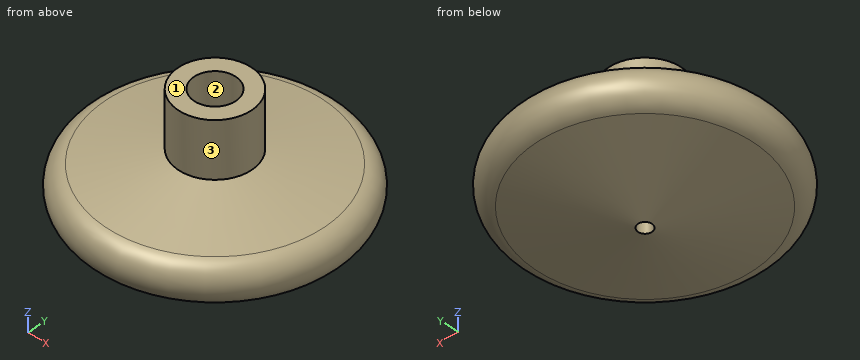
from build123d import *

# Parameters (mm, degrees)
F2_R     = 4.7625
F3_DEPTH = 9.525
F4_R     = 1.5875
F5_DEPTH = 12.7


with BuildPart() as f1:
    # F0 (on Front) → F1 (revolve)
    with BuildSketch(Plane.XZ):
        with BuildLine():
            Line((0, 29.8668724909), (0, 0))
            Line((0, 0), (24.9306534148, 4.8691192822))
            ThreePointArc((24.9306534148, 4.8691192822), (28.6638483422, 9.4019658913), (24.9306534148, 13.9348125005))
            Line((24.9306534148, 13.9348125005), (8.382, 17.1668724909))
            Line((8.382, 17.1668724909), (8.382, 29.8668724909))
            Line((8.382, 29.8668724909), (0, 29.8668724909))
        make_face()
    revolve(axis=Axis((0, 0, 14.9334362454), (0, 0, -1)))

    # F2 (on face) → F3 (cut)
    with BuildSketch(Plane.XY.offset(29.8668724909)):
        Circle(F2_R)
    extrude(amount=-F3_DEPTH, mode=Mode.SUBTRACT)

    # F4 (on Top) → F5 (cut)
    with BuildSketch(Plane.XY):
        Circle(F4_R)
    extrude(amount=F5_DEPTH, mode=Mode.SUBTRACT)


solid = f1.part
Check sheet for the modelled part. Datum: model origin and axes. Units: mm. Face numbers are marked on the shaded views. Round coordinates to 2 decimals unless told otherwise and drop trailing zeros. Write each loop counter-clockwise with the first axis right and the second up, starting at its lowest first coordinate (ties: lowest second). Pieces come first, ordered by that corner, then holes. Notation, with made-up numbers: (57.5, 63) - (61.5, 63) arc R15 ccw to (61.5, 88) - close; hole circle Ø2 at (-27.5, -0.5). An arc over 180 degrees is marked (long way). Return JSON: item names as keys, results as strings.
Q1. Scan lines: L1, parallel to Y at x = 0, z = 25.5; L2, parallel to Y at x = 0, z = 9.5; L3, parallel to X at y = 0, z = 5.5. Record each from-to range of solid material in increasing order. Write a range as from..to.
Returned:
{"L1": "y = -8.38..-4.76, 4.76..8.38", "L2": "y = -28.66..-1.59, 1.59..28.66", "L3": "x = -26.52..-1.59, 1.59..26.52"}
Q2. Draft check along X on the marked faces 1, 2 and 3. Enter one of: released by +X, released by -X, zero draft, split by the parting line, or undercut.
Returned:
{"face 1": "zero draft", "face 2": "undercut", "face 3": "split by the parting line"}
Q3. Cross-section at A-A (y = 0). Record the boundary of the cut face in (x, z).
Returned:
{"outline": "(-24.93, 4.87) - (-1.59, 0.31) - (-1.59, 12.7) - (1.59, 12.7) - (1.59, 0.31) - (24.93, 4.87) arc R4.62 ccw to (24.93, 13.93) - (8.38, 17.17) - (8.38, 29.87) - (4.76, 29.87) - (4.76, 20.34) - (-4.76, 20.34) - (-4.76, 29.87) - (-8.38, 29.87) - (-8.38, 17.17) - (-24.93, 13.93) arc R4.62 ccw to start"}
Q4. Depth check by flat-ended pin: P1, Ø1, axis at x = -20, z = 8, coming from the +Y side; P2, Ø1, axis at x = -0.5, y = 0.5, coming from the -Z side; P3, Ø3, axis at x = -0.5, y = -0.5, coming from the +Z side. Enter the tip coordinate at first touch or a pass-through.
Returned:
{"P1": "stops at y = 20.75", "P2": "stops at z = 12.7", "P3": "stops at z = 20.34"}
Q5. Cross-section at D-D (z = 16.25). Record the boundary of the cut face in (x, y).
Returned:
{"outline": "circle Ø26.15 at (0, 0)"}
Q6. Cross-section at B-B (z = 26). Record the boundary of the cut face in (x, y) (1 decimal), then the cut area to 3 significant figures.
Returned:
{"outline": "circle Ø16.8 at (0, 0); hole circle Ø9.5 at (0, 0)", "area": "149 mm²"}
